from build123d import *

# Parameters (mm, degrees)
EXTRUDE_2_DEPTH          = 8
EXTRUDE_4_DEPTH          = 3
CUT_EXTRUDE_2_DEPTH      = 121.7683733433551
CUT_EXTRUDE_2_DEPTH_BACK = 121.7683733433551
CUT_EXTRUDE_3_DEPTH      = 121.7683733433551
CUT_EXTRUDE_3_DEPTH_BACK = 121.7683733433551
SKETCH_7_R               = 1.6000000000000003
SKETCH_8_R               = 1.2500000000000009
CUT_EXTRUDE_4_DEPTH      = 121.7683733433551
PATTERN_LINEAR_1_COUNT   = 7
PATTERN_LINEAR_1_PITCH   = 10
SKETCH_9_W               = 25
SKETCH_9_H               = 20.00000000000002
EXTRUDE_5_DEPTH          = 4
SKETCH_10_W              = 23
SKETCH_10_H              = 17
EXTRUDE_7_DEPTH          = 1


with BuildPart() as part:
    # Sketch 5 → Extrude 2 (new, symmetric)
    with BuildSketch(Plane.XY):
        with BuildLine():
            Line((-8, -7.5498344352708955), (-8, 7.5498344352708955))
            ThreePointArc((-7.999999999999892, 7.549834435270865), (-11, 1.35e-15), (-7.9999999999998925, -7.5498344352708635))
        make_face()
        with BuildLine():
            Line((0, 4.050000000000001), (0, 11))
            ThreePointArc((-1.9228e-13, 11), (-4.35613482413148, 10.100697470669488), (-7.999999999999892, 7.549834435270865))
            Line((-8, 7.5498344352708955), (-8, -7.5498344352708955))
            ThreePointArc((-7.9999999999998925, -7.5498344352708635), (-4.356134824131392, -10.100697470669525), (-2.02e-15, -11))
            Line((0, -11.000000000000004), (0, -4.050000000000001))
            ThreePointArc((-5.47e-14, -4.05), (-4.05, 5e-16), (-5.191e-14, 4.05))
        make_face()
        with BuildLine():
            ThreePointArc((8.00000000000005, 7.549834435270696), (4.356134824131412, 10.100697470669518), (-1.9228e-13, 11))
            Line((0, 11), (0, 4.050000000000001))
            ThreePointArc((-5.191e-14, 4.05), (2.863782463805499, 2.8637824638055354), (4.05, 0))
            ThreePointArc((4.05, -9.9e-16), (2.863782463805499, -2.863782463805536), (-5.47e-14, -4.05))
            Line((0, -4.050000000000001), (0, -11.000000000000004))
            ThreePointArc((-2.02e-15, -11), (4.356134824131496, -10.10069747066948), (8.000000000000048, -7.549834435270699))
            Line((8, -7.549834435270682), (8, 7.549834435270682))
        make_face()
        with BuildLine():
            ThreePointArc((11, 0), (10.22252415013045, 4.062019202317946), (8.00000000000005, 7.549834435270696))
            Line((8, 7.549834435270682), (8, -7.549834435270682))
            ThreePointArc((8.000000000000048, -7.549834435270699), (10.222524150130448, -4.062019202317949), (11, -2.69e-15))
        make_face()
    extrude(amount=EXTRUDE_2_DEPTH, both=True)

    # Sketch 5_5 → Extrude 4 (add, symmetric)
    with BuildSketch(Plane.XY):
        with BuildLine():
            Line((-8, -7.5498344352708955), (-8, -120))
            Line((-8, -120), (8, -120))
            Line((8, -120), (8, -7.549834435270682))
            ThreePointArc((8.000000000000048, -7.549834435270699), (1.1522e-13, -11), (-7.9999999999998925, -7.5498344352708635))
        make_face()
    extrude(amount=EXTRUDE_4_DEPTH, both=True)

    # Sketch 6 → Cut-Extrude 2 (cut, two sides: drawn at the far end of the back side and taken through both)
    with BuildSketch(Plane.XY.offset(-CUT_EXTRUDE_2_DEPTH_BACK)):
        Polygon((-0.7500000000000006, -3), (0.7499999999999994, -2.9999999999999996), (0.7500000000000013, -15), (-0.7499999999999987, -15), align=None)
    extrude(amount=CUT_EXTRUDE_2_DEPTH + CUT_EXTRUDE_2_DEPTH_BACK, mode=Mode.SUBTRACT)

    # Sketch 7 → Cut-Extrude 3 (cut, two sides: drawn at the far end of the back side and taken through both)
    with BuildSketch(Plane(origin=(0, 0, 0), x_dir=(0, 0, -1), z_dir=(1, 0, 0)).offset(-CUT_EXTRUDE_3_DEPTH_BACK)):
        with Locations(Location((0, -12, 0), (0, 0, 270))):
            Circle(SKETCH_7_R)
    extrude(amount=CUT_EXTRUDE_3_DEPTH + CUT_EXTRUDE_3_DEPTH_BACK, mode=Mode.SUBTRACT)

    # Sketch 8 → Cut-Extrude 4 (cut, symmetric)
    with BuildSketch(Plane.XY):
        with Locations((4.9e-15, -40)):
            Circle(SKETCH_8_R)
    cut_extrude_4 = extrude(amount=CUT_EXTRUDE_4_DEPTH, both=True, mode=Mode.SUBTRACT)

    # Pattern Linear 1: Cut-Extrude 4 ×7
    with Locations(*[(0, -i * PATTERN_LINEAR_1_PITCH, 0) for i in range(1, PATTERN_LINEAR_1_COUNT)]):
        add(cut_extrude_4, mode=Mode.SUBTRACT)

    # Sketch 9 → Extrude 5 (add)
    with BuildSketch(Plane.XZ.offset(120)):
        Rectangle(SKETCH_9_W, SKETCH_9_H)
    extrude(amount=EXTRUDE_5_DEPTH)

    # Sketch 10 → Extrude 7 (add)
    with BuildSketch(Plane.XZ.offset(124)):
        Polygon((-13.5, -10.5), (-13.5, 10.5), (13.5, 10.500000000000002), (13.500000000000002, -10.5), align=None)
        Rectangle(SKETCH_10_W, SKETCH_10_H, mode=Mode.SUBTRACT)
    extrude(amount=EXTRUDE_7_DEPTH)


solid = part.part
Geometry check sheet. Reference: the model listing, model coordinates, mm. A direction names the side the tool comes from. Coordinates: 2 decimals unless noted, no trailing zeros. Order: outer loops, then holes, each group sorted by start corner. A loop starts at its lowest first (then second) coordinate and runs counter-clockwise, first axis right, second up. Notation, with made-up numbers: (29.5, -38.5) - (74.5, -38.5) arc R14 ccw to (74.5, -15.5) - close; hole circle Ø11 at (-28.5, 60). An arc over 180 degrees is marked (long way). Answer in a Markdown table with one row per item. Add a question column.
1) Gauge pin test, flat ends, axial feed: P1, Ø6.5, axis at y = -80.5, z = -1.5, coming from the -X side; P2, Ø3, axis at x = 0, y = -80, coming from the +Z side; P3, Ø3, axis at x = -5.5, z = -2, coming from the +Y side. Record the tip position at first contact, or that the pin passes through.
2) Cross-section at C-C, the plane z = 0. State how many separate pieces and enclosed holes the cut face has, then the cut area to 3 significant figures.
3) Cross-section at D-D, the plane y = -90. Record the cut outline in (x, z), then the cut area to 3 significant figures.
4) Cross-section at A-A, the plane y = 0. Record the cut outline in (x, z).
5) Cross-section at B-B, the plane z = 5.75. Record the cut outline in (x, y), then the cut area to 3 significant figures.
6) Material ranges on line 1 along Y through (x, z) = (-3, -0.25); line 2 along X through (y, z) = (-113, 0.75); line 3 along Y through (x, z) = (-12, 2), recorded low to high. Write a range as [from, to].
7) Release check for a two-part mould opening along Y. For faces 4 (the flat face through (-12.5, -122, 0)), 5 (the flat face through (0, -120, 5)), 6 (the flat face through (0, -125, -9)) record: +Y half, -Y half, draft (parallel to the pull), parting line (faces both ways), or undercut.
8) Set-up check for faces 1 (the flat face through (8, -65, 0)), 2 (the flat face through (0, -122, 10)), 3 (the flat face through (12.5, -122, 0)): record each of +Z, -Z, +X, -X, +Y, -Y from which the full face is reachable in a straight line by a thin tool's end or side.
Check result:
| question | item | result |
|---|---|---|
| 1 | P1 | stops at x = -8 |
| 1 | P2 | stops at z = 3 |
| 1 | P3 | stops at y = 10.25 |
| 2 | separate pieces | 2 |
| 2 | enclosed holes | 7 |
| 2 | area | 2,100 mm² |
| 3 | outline | (-8, -3) - (-1.25, -3) - (-1.25, 3) - (-8, 3) - close; (1.25, -3) - (8, -3) - (8, 3) - (1.25, 3) - close |
| 3 | area | 81.0 mm² |
| 4 | outline | (-11, -8) - (-4.05, -8) - (-4.05, 8) - (-11, 8) - close; (4.05, -8) - (11, -8) - (11, 8) - (4.05, 8) - close |
| 5 | outline | (-13.5, -125) - (-11.5, -125) - (-11.5, -124) - (11.5, -124) - (11.5, -125) - (13.5, -125) - (13.5, -124) - (12.5, -124) - (12.5, -120) - (-12.5, -120) - (-12.5, -124) - (-13.5, -124) - close; (-0.75, -10.97) - (-0.75, -3.98) arc R4.05 cw (long way) to (0.75, -3.98) - (0.75, -10.97) arc R11 ccw (long way) to start |
| 5 | area | 422 mm² |
| 6 | line 1 | y = [-124, -13.58], [-10.42, -2.72], [2.72, 10.58] |
| 6 | line 2 | x = [-8, 8] |
| 6 | line 3 | y = [-125, -120] |
| 7 | face 4 | draft |
| 7 | face 5 | undercut |
| 7 | face 6 | -Y half |
| 8 | face 1 | +Z, -Z, +X |
| 8 | face 2 | +Z, +X, -X, +Y |
| 8 | face 3 | +Z, -Z, +X, +Y |
